```python
from build123d import *

# Parameters (mm, degrees)
F0_W     = 59.5
F0_H     = 59.5
F1_DEPTH = 15.3
F2_R     = 2.125
F3_DEPTH = 25


with BuildPart() as f1:
    # F0 (on Right) → F1 (new body)
    with BuildSketch(Plane.YZ):
        Rectangle(F0_W, F0_H)
        with BuildLine():
            ThreePointArc((-2.920188, -28.35), (-20.152543, -20.152543), (-28.35, -2.920188))
            Line((-28.35, -2.920188), (-28.35, 2.920188))
            ThreePointArc((-28.35, 2.920188), (-20.152543, 20.152543), (-2.920188, 28.35))
            Line((-2.920188, 28.35), (2.920188, 28.35))
            ThreePointArc((2.920188, 28.35), (20.152543, 20.152543), (28.35, 2.920188))
            Line((28.35, 2.920188), (28.35, -2.920188))
            ThreePointArc((28.35, -2.920188), (20.152543, -20.152543), (2.920188, -28.35))
            Line((2.920188, -28.35), (-2.920188, -28.35))
        make_face(mode=Mode.SUBTRACT)
    extrude(amount=F1_DEPTH)

    # F2 (on face) → F3 (cut)
    with BuildSketch(Plane.YZ.offset(15.3)):
        with Locations((-24.875, 24.875)):
            Circle(F2_R)
        with Locations((24.875, 24.875)):
            Circle(F2_R)
        with Locations((24.875, -24.875)):
            Circle(F2_R)
        with Locations((-24.875, -24.875)):
            Circle(F2_R)
    extrude(amount=-F3_DEPTH, mode=Mode.SUBTRACT)


solid = f1.part
```
CAD build for the part. Positions are in the model's coordinates, mm. A direction names the side the tool comes from. Round coordinates to 2 decimals unless told otherwise and drop trailing zeros. Write each loop counter-clockwise with the first axis right and the second up, starting at its lowest first coordinate (ties: lowest second). Pieces come first, ordered by that corner, then holes.
Item 1: Mould opens along Y. For faces 3 (the cylindrical face through (7.543, 20.344, -19.959)), 4 (the flat face through (8, 29.75, 0)), 5 (the flat face through (8, 0, 29.75)), 6 (the cylindrical face through (7.76, 23.19, 23.58)) say: released by +Y, released by -Y, zero draft, split by the parting line, or undercut.
Filled in:
face 3: undercut
face 4: released by +Y
face 5: zero draft
face 6: undercut
Item 2: Drop a flat-ended pin along its axis: pin 1 Ø3.5 at (y, z) = (-24.875, -24.875) entering from +X. Give the stop position or say it passes through.
Filled in:
pin 1: passes through
Item 3: Tool access for faces 1 (the flat face through (8, 0, -29.75)), 2 (the cylindrical face through (7.543, -19.959, -20.344)): list every direction of +Z, -Z, +X, -X, +Y, -Y with a clear straight run to the whole face (end or side of a thin tool).
Filled in:
face 1: -Z, +X, -X, +Y, -Y
face 2: +X, -X
Item 4: Band-saw the part on B-B on z = 13. Write the cut outline in (x, y).
Filled in:
outline: (0, -29.75) - (15.3, -29.75) - (15.3, -25.36) - (0, -25.36) - close; (0, 25.36) - (15.3, 25.36) - (15.3, 29.75) - (0, 29.75) - close
Item 5: Band-saw the part on A-A on y = -14.5. Write the cut outline in (x, z), then the cut area to 3 significant figures.
Filled in:
outline: (0, -29.75) - (15.3, -29.75) - (15.3, -24.54) - (0, -24.54) - close; (0, 24.54) - (15.3, 24.54) - (15.3, 29.75) - (0, 29.75) - close
area: 160 mm2
Item 6: Band-saw the part on C-C on x = 8.5. Write the cut outline in (y, z) (3 decimals).
Filled in:
outline: (-29.75, -29.75) - (29.75, -29.75) - (29.75, 29.75) - (-29.75, 29.75) - close; hole (-28.35, -2.92) arc R28.5 ccw to (-2.92, -28.35) - (2.92, -28.35) arc R28.5 ccw to (28.35, -2.92) - (28.35, 2.92) arc R28.5 ccw to (2.92, 28.35) - (-2.92, 28.35) arc R28.5 ccw to (-28.35, 2.92) - close; hole circle Ø4.25 at (-24.875, -24.875); hole circle Ø4.25 at (-24.875, 24.875); hole circle Ø4.25 at (24.875, -24.875); hole circle Ø4.25 at (24.875, 24.875)
Item 7: Drill centre lines: L1, parallel to Y at x = 4, z = 2.5; L2, parallel to Z at x = 9, y = 11. Where is each one in solid material? Low to high.
Filled in:
L1: y = -29.75 to -28.35, 28.35 to 29.75
L2: z = -29.75 to -26.29, 26.29 to 29.75
Item 8: Band-saw the part on D-D on y = -25.5. Write the cut outline in (x, z).
Filled in:
outline: (0, -29.75) - (15.3, -29.75) - (15.3, -26.91) - (0, -26.91) - close; (0, -22.84) - (15.3, -22.84) - (15.3, -12.73) - (0, -12.73) - close; (0, 12.73) - (15.3, 12.73) - (15.3, 22.84) - (0, 22.84) - close; (0, 26.91) - (15.3, 26.91) - (15.3, 29.75) - (0, 29.75) - close
